Geometry check sheet. Reference: the model listing, model coordinates, mm. A direction names the side the tool comes from. Coordinates: 2 decimals unless noted, no trailing zeros. Write each loop counter-clockwise with the first axis right and the second up, starting at its lowest first coordinate (ties: lowest second). Pieces come first, ordered by that corner, then holes. Notation, with made-up numbers: (74.25, 55.5) -> (87.25, 55.5) arc R26 cw to (87.25, 71.5) -> close; hole circle Ø5 at (-31.5, -29.5). An arc over 180 degrees is marked (long way). Use a Markdown table: item, result.
```python
from build123d import *

# Parameters (mm, degrees)
SKETCH5_W = 3.2385
SKETCH5_H = 3.81


with BuildPart() as part:
    # Sketch1 → Revolve1 (revolve)
    with BuildSketch(Plane.XY):
        with BuildLine():
            Line((0, 0), (0, 4.8006))
            Line((0, 4.8006), (0.75565, 5.55625))
            Line((0.75565, 5.55625), (5.028593864, 5.55625))
            Line((5.028593864, 5.55625), (5.786403291, 4.804192648))
            ThreePointArc((5.786403291, 4.804192648), (6.045223575, 4.6323221), (6.35, 4.572))
            Line((6.35, 4.572), (7.5184, 4.572))
            ThreePointArc((7.5184, 4.572), (8.084156136, 4.806343864), (8.3185, 5.3721))
            Line((8.3185, 5.3721), (8.3185, 5.5245))
            Line((8.3185, 5.5245), (9.525, 5.5245))
            Line((9.525, 5.5245), (9.525, 0))
            Line((9.525, 0), (0, 0))
        make_face()
    revolve(axis=Axis((9.525, 0, 0), (-1, 0, 0)))

    # Sketch2 → Revolve2 (revolve)
    with BuildSketch(Plane.XY):
        Polygon((9.525, 0), (9.525, 9.3726), (25.4, 9.3726), (25.4, 5.16255), (25.908, 5.16255), (26.416, 5.67055), (29.6672, 5.67055), (30.1752, 5.16255), (30.1752, 0), align=None)
    revolve(axis=Axis((30.1752, 0, 0), (-1, 0, 0)))

    # Sketch3 → Cut-Revolve1 (revolve, cut)
    with BuildSketch(Plane.XY):
        Polygon((0, 0), (0, 2.91465), (0.508, 2.40665), (30.1752, 2.40665), (30.1752, 0), align=None)
    revolve(axis=Axis((30.1752, 0, 0), (-1, 0, 0)), mode=Mode.SUBTRACT)

    # Sketch4 → Cut-Revolve2 (revolve, cut)
    with BuildSketch(Plane(origin=(0, 0, 0), x_dir=(1, 0, 0), z_dir=(0, 1, 0))):
        Polygon((18.288, 1.016), (20.27174, 1.016), (20.27174, -7.92734), (20.701, -8.3566), (22.2504, -8.3566), (22.2504, -9.3726), (18.288, -9.3726), align=None)
    revolve(axis=Axis((18.288, 0, 9.3726), (0, 0, -1)), mode=Mode.SUBTRACT)

    # Sketch5 → Cut-Revolve3 (revolve, cut)
    with BuildSketch(Plane.XY):
        with Locations((23.78075, 8.07085)):
            Rectangle(SKETCH5_W, SKETCH5_H)
    revolve(axis=Axis((25.4, 0, 0), (-1, 0, 0)), mode=Mode.SUBTRACT)

    # Sketch6 → Revolve3 (revolve)
    with BuildSketch(Plane.XY):
        with BuildLine():
            Line((25.4, 5.660338686), (25.4, 4.90855))
            Line((25.4, 4.90855), (25.908, 4.90855))
            Line((25.908, 4.90855), (25.908, 5.16255))
            Line((25.908, 5.16255), (25.654, 5.16255))
            Line((25.654, 5.16255), (25.511592316, 5.304957684))
            ThreePointArc((25.511592316, 5.304957684), (25.474394878, 5.394760245), (25.511592316, 5.484562806))
            Line((25.511592316, 5.484562806), (26.108711314, 6.081681804))
            Line((26.108711314, 6.081681804), (26.108711314, 6.16585))
            Line((26.108711314, 6.16585), (25.905511314, 6.16585))
            Line((25.905511314, 6.16585), (25.4, 5.660338686))
        make_face()
    revolve(axis=Axis((25.908, 0, 0), (-1, 0, 0)))


solid = part.part
```
Item 1: Depth check by flat-ended pin: P1, Ø1, axis at x = 22, y = -5, coming from the -Z side; P2, Ø6.5, axis at x = 18.288, y = 0, coming from the +Z side; P3, Ø2, axis at x = 14, z = -6.5, coming from the -Y side. Enter the tip coordinate at first touch or a pass-through.
Answer block:
| item | result |
|---|---|
| P1 | stops at z = -8.22 |
| P2 | stops at z = 8.36 |
| P3 | stops at y = -7.59 |
Item 2: Section check B-B on y = 0. Count the separate pieces of the cut face and the enclosed holes in it, then the cut area to 3 significant figures.
Answer block:
| item | result |
|---|---|
| separate pieces | 3 |
| enclosed holes | 0 |
| area | 253 mm^2 |
Item 3: Section check A-A on x = 7. Record the boundary of the cut face in (y, z).
Answer block:
| item | result |
|---|---|
| outline | circle Ø9.14 at (0, 0); hole circle Ø4.81 at (0, 0) |
Item 4: Thickness scan on L1, parallel to Z at x = 21.75, y = 0; L2, parallel to X at y = -4.25, z = 3; L3, parallel to X at y = 2, z = -8.25 (1 decimal). Record the ranges inside material, lowest first. Write a range as [from, to].
Answer block:
| item | result |
|---|---|
| L1 | z = [-9.37, -2.41], [2.41, 8.36] |
| L2 | x = [0.4, 5.39], [8.3, 25.61], [25.95, 30.14] |
| L3 | x = [9.5, 22.2] |
Item 5: Tool access check on faces 4 (the flat face through (30.175, 1.1, -2.4)), 5 (the cylindrical face through (8.93, -0.719, -5.477)), 6 (the cylindrical face through (14.33, -0.16, 8.76)). Record the directions out of +Z, -Z, +X, -X, +Y, -Y that give a thin tool (end or side, any length) a straight path to the whole face; none if there is none.
Answer block:
| item | result |
|---|---|
| face 4 | +Z, -Z, +X, +Y, -Y |
| face 5 | none |
| face 6 | +Z |
Item 6: Mould release check, pull along X, two halves, no side actions. Record for faces 1 (the flat face through (22.162, -2, 6)), 2 (the cylindrical face through (2.92, 5.3, -1.67)), 3 (the cylindrical face through (20, 1, 5)): +X half, -X half, draft (parallel to the pull), parting line (faces both ways), or undercut.
Answer block:
| item | result |
|---|---|
| face 1 | +X half |
| face 2 | draft |
| face 3 | undercut |
Item 7: Section check D-D on y = -8. Record the boundary of the cut face in (x, z) (1 decimal), then the cut area to 3 significant figures.
Answer block:
| item | result |
|---|---|
| outline | (9.5, -4.9) -> (22.2, -4.9) -> (22.2, 4.9) -> (9.5, 4.9) -> close |
| area | 123 mm^2 |
Item 8: Section check C-C on z = -7. Record the boundary of the cut face in (x, y) (1 decimal).
Answer block:
| item | result |
|---|---|
| outline | (9.5, -6.2) -> (22.2, -6.2) -> (22.2, 6.2) -> (9.5, 6.2) -> close |
